Work out the finished part from the listing and answer in its coordinate system (mm). A direction names the side the tool comes from. Round coordinates to 2 decimals unless told otherwise and drop trailing zeros. Write each loop counter-clockwise with the first axis right and the second up, starting at its lowest first coordinate (ties: lowest second). Pieces come first, ordered by that corner, then holes.
from build123d import *

# Parameters (mm, degrees)
SKETCH1_W           = 430
SKETCH1_H           = 500
BOSS_EXTRUDE1_DEPTH = 1.5
SKETCH2_W           = 48.6
SKETCH2_H           = 75
CUT_EXTRUDE1_DEPTH  = 10
SKETCH3_W           = 35
SKETCH3_H           = 450
CUT_EXTRUDE2_DEPTH  = 10
CUT_EXTRUDE3_DEPTH  = 10
FILLET2_R           = 2
FILLET3_R           = 2
SKETCH6_R           = 2
CUT_EXTRUDE4_DEPTH  = 10


with BuildPart() as part:
    # Sketch1 → Boss-Extrude1 (new body)
    with BuildSketch(Plane(origin=(0, 0, 0), x_dir=(1, 0, 0), z_dir=(0, 1, 0))):
        with Locations((6126.084066999, -8702.312377786)):
            Rectangle(SKETCH1_W, SKETCH1_H)
    extrude(amount=BOSS_EXTRUDE1_DEPTH)

    # Sketch2 → Cut-Extrude1 (cut)
    with BuildSketch(Plane(origin=(0, 1.5, 0), x_dir=(1, 0, 0), z_dir=(0, 1, 0))):
        with Locations((5935.384066999, -8644.812377786)):
            Rectangle(SKETCH2_W, SKETCH2_H)
        with Locations((6316.784066999, -8644.812377786)):
            Rectangle(SKETCH2_W, SKETCH2_H)
    extrude(amount=-CUT_EXTRUDE1_DEPTH, mode=Mode.SUBTRACT)

    # Sketch3 → Cut-Extrude2 (cut)
    with BuildSketch(Plane(origin=(0, 1.5, 0), x_dir=(1, 0, 0), z_dir=(0, 1, 0))):
        Polygon((5969.084066999, -8541.651929061), (5969.084066999, -8927.312377786), (6004.084066999, -8927.312377786), (6004.084066999, -8477.312377786), (5969.084066999, -8477.312377786), align=None)
        with Locations((6265.584066999, -8702.312377786)):
            Rectangle(SKETCH3_W, SKETCH3_H)
        Polygon((6102.084066999, -8487.312377786), (6136.084066999, -8487.312377786), (6136.084066999, -8917.312377786), (6111.084066999, -8917.312377786), (6111.084066999, -8532.312377786), (6066.084066999, -8532.312377786), (6066.084066999, -8487.312377786), align=None)
    extrude(amount=-CUT_EXTRUDE2_DEPTH, mode=Mode.SUBTRACT)

    # Sketch4 → Cut-Extrude3 (cut)
    with BuildSketch(Plane(origin=(0, 1.5, 0), x_dir=(1, 0, 0), z_dir=(0, 1, 0))):
        with BuildLine():
            Line((6234.584067167, -8840.596520357), (6177.084066999, -8898.096518708))
            Line((6177.084066999, -8898.096518708), (6174.584066999, -8900.596520951))
            ThreePointArc((6174.584066999, -8900.596520951), (6174.584069168, -8905.596518633), (6179.584066849, -8905.596518637))
            Line((6179.584066849, -8905.596518637), (6237.084067092, -8848.09652021))
            Line((6237.084067092, -8848.09652021), (6239.584067017, -8845.596520364))
            ThreePointArc((6239.584067017, -8845.596520364), (6239.584067096, -8840.596520436), (6234.584067167, -8840.596520357))
        make_face()
        with BuildLine():
            ThreePointArc((6174.584067387, -8880.596519018), (6174.584067598, -8885.596518612), (6179.584067193, -8885.596518982))
            Line((6179.584067193, -8885.596518982), (6229.584067988, -8835.596519766))
            ThreePointArc((6229.584067988, -8835.596519766), (6229.584069287, -8830.596518949), (6224.584068469, -8830.596519802))
            Line((6224.584068469, -8830.596519802), (6222.084069197, -8833.096518708))
            Line((6222.084069197, -8833.096518708), (6174.584067387, -8880.596519018))
        make_face()
        with BuildLine():
            ThreePointArc((6174.584067774, -8860.596519406), (6174.584068372, -8865.596518614), (6179.58406758, -8865.59651937))
            Line((6179.58406758, -8865.59651937), (6209.58406806, -8835.596519838))
            ThreePointArc((6209.58406806, -8835.596519838), (6209.584069287, -8830.596518805), (6204.584068253, -8830.596519874))
            Line((6204.584068253, -8830.596519874), (6174.584067774, -8860.596519406))
        make_face()
        with BuildLine():
            Line((6219.584066911, -8905.596518637), (6239.584067017, -8885.596519163))
            ThreePointArc((6239.584067017, -8885.596519163), (6239.584067096, -8880.596519234), (6234.584067167, -8880.596519155))
            Line((6234.584067167, -8880.596519155), (6214.584067061, -8900.596518629))
            ThreePointArc((6214.584067061, -8900.596518629), (6214.584066907, -8905.596518633), (6219.584066911, -8905.596518637))
        make_face()
        with BuildLine():
            ThreePointArc((6174.584068161, -8840.596519795), (6174.584069146, -8845.596518616), (6179.584067967, -8845.596519759))
            Line((6179.584067967, -8845.596519759), (6189.584068132, -8835.59651991))
            ThreePointArc((6189.584068132, -8835.59651991), (6189.584069431, -8830.596518805), (6184.584068325, -8830.596519946))
            Line((6184.584068325, -8830.596519946), (6174.584068161, -8840.596519795))
        make_face()
        with BuildLine():
            Line((6234.584067693, -8860.59651923), (6194.58406703, -8900.596518629))
            ThreePointArc((6194.58406703, -8900.596518629), (6194.584066876, -8905.596518633), (6199.58406688, -8905.596518637))
            Line((6199.58406688, -8905.596518637), (6237.084067092, -8868.096519609))
            Line((6237.084067092, -8868.096519609), (6239.584067543, -8865.596517133))
            ThreePointArc((6239.584067543, -8865.596517133), (6239.584066044, -8860.596518783), (6234.584067693, -8860.59651923))
        make_face()
        with BuildLine():
            Line((6237.084067092, -8898.096518708), (6234.584067092, -8900.596518629))
            ThreePointArc((6234.584067092, -8900.596518629), (6233.817659407, -8904.449508447), (6237.084067092, -8906.632051027))
            Line((6237.084067092, -8906.632051027), (6237.084067092, -8898.096518708))
        make_face()
    extrude(amount=-CUT_EXTRUDE3_DEPTH, mode=Mode.SUBTRACT)

    # Fillet2
    fillet2_edges = [part.edges().sort_by_distance(p)[0] for p in [
        (5959.684066999, 0.75, 8607.312377786),
        (5959.684066999, 0.75, 8682.312377786),
        (5911.084066999, 0.75, 8682.312377786),
        (5911.084066999, 0.75, 8607.312377786),
        (6341.084066999, 0.75, 8607.312377786),
        (6341.084066999, 0.75, 8682.312377786),
        (6292.484066999, 0.75, 8682.312377786),
        (6292.484066999, 0.75, 8607.312377786),
        (5911.084066999, 0.75, 8452.312377786),
        (6341.084066999, 0.75, 8452.312377786),
        (6341.084066999, 0.75, 8952.312377786),
        (5911.084066999, 0.75, 8952.312377786),
    ]]
    fillet(fillet2_edges, radius=FILLET2_R)

    # Fillet3
    fillet3_edges = [part.edges().sort_by_distance(p)[0] for p in [
        (6283.084066999, 0.75, 8477.312377786),
        (6283.084066999, 0.75, 8927.312377786),
        (6248.084066999, 0.75, 8927.312377786),
        (6248.084066999, 0.75, 8477.312377786),
        (5969.084066999, 0.75, 8477.312377786),
        (6004.084066999, 0.75, 8477.312377786),
        (6004.084066999, 0.75, 8927.312377786),
        (5969.084066999, 0.75, 8927.312377786),
        (6066.084066999, 0.75, 8532.312377786),
        (6066.084066999, 0.75, 8487.312377786),
        (6136.084066999, 0.75, 8487.312377786),
        (6136.084066999, 0.75, 8917.312377786),
        (6111.084066999, 0.75, 8917.312377786),
        (6111.084066999, 0.75, 8532.312377786),
    ]]
    fillet(fillet3_edges, radius=FILLET3_R)

    # Sketch6 → Cut-Extrude4 (cut)
    with BuildSketch(Plane(origin=(0, 1.5, 0), x_dir=(1, 0, 0), z_dir=(0, 1, 0))):
        with Locations((6212.584066999, -8822.590833806)):
            Circle(SKETCH6_R)
        with Locations((6212.584066999, -8917.590833806)):
            Circle(SKETCH6_R)
        with Locations((6167.584066999, -8865.596518708)):
            Circle(SKETCH6_R)
    extrude(amount=-CUT_EXTRUDE4_DEPTH, mode=Mode.SUBTRACT)


solid = part.part
Q1. Find the intervals of material crossed by L1, parallel to X at y = 0.75, z = 8552; L2, parallel to X at y = 0.6, z = 8484.5; L3, parallel to Z at x = 5987.5, y = 0.25, in increasing order.
Q2. Find section A-A (z = 8636). Determine the outline of the cut face in (x, y).
Q3. Find section C-C (y = 0.9). Count the separate pieces of the cut face and the enclosed holes in it, plus the area to 3 significant figures.
Q4. A tool of negligible diameter and unlimited length cuts with its end or side. For faces 1 (the face through (6184.51, 0.76, 8840.67)), 2 (the face through (6075, 1.5, 8699)), from which of +Z, -Z, +X, -X, +Y, -Y can it reach the whole face along a straight path? Write none if from no direction.
Q5. Given pin 1 (12 mm diameter, centred on x = 5962.5, z = 8574.5, fed in from -Y); pin 2 (0.8 mm diameter, centred on y = 0.5, z = 8636, fed in from -X), each flat-ended and moving along its own axis, determine where each tip first touches the part or whether it passes through.
Q6. Find section B-B (z = 8783). Determine the outline of the cut face in (x, y), plus the area to 4 significant figures.
Q7. The mould has two halves that part along Z. Classify faces 3 (the face through (6075, 0, 8699)), 4 (the face through (6224.72, 0.76, 8890.46)): +Z half, -Z half, draft (parallel to the pull), parting line (faces both ways), or undercut.
Report:
1. L1: x = 5911.08 to 5969.08, 6004.08 to 6111.08, 6136.08 to 6248.08, 6283.08 to 6341.08
1. L2: x = 5911.08 to 5969.08, 6004.08 to 6248.08, 6283.08 to 6341.08
1. L3: z = 8452.31 to 8477.31, 8927.31 to 8952.31
2. outline: (5959.68, 0) - (5969.08, 0) - (5969.08, 1.5) - (5959.68, 1.5) - close; (6004.08, 0) - (6111.08, 0) - (6111.08, 1.5) - (6004.08, 1.5) - close; (6136.08, 0) - (6248.08, 0) - (6248.08, 1.5) - (6136.08, 1.5) - close; (6283.08, 0) - (6292.48, 0) - (6292.48, 1.5) - (6283.08, 1.5) - close
3. separate pieces: 1
3. enclosed holes: 13
3. area: 161,000 mm2
4. face 1: +Y, -Y
4. face 2: +Z, -Z, +X, -X, +Y
5. pin 1: stops at y = 0
5. pin 2: stops at x = 5959.68
6. outline: (5911.08, 0) - (5969.08, 0) - (5969.08, 1.5) - (5911.08, 1.5) - close; (6004.08, 0) - (6111.08, 0) - (6111.08, 1.5) - (6004.08, 1.5) - close; (6136.08, 0) - (6248.08, 0) - (6248.08, 1.5) - (6136.08, 1.5) - close; (6283.08, 0) - (6341.08, 0) - (6341.08, 1.5) - (6283.08, 1.5) - close
6. area: 502.5 mm2
7. face 3: draft
7. face 4: undercut
